```python
from build123d import *

# Parameters (mm, degrees)
BOSS_EXTRUDE1_DEPTH = 6.35
SKETCH2_W           = 71.12
SKETCH2_H           = 9.525
CUT_EXTRUDE1_DEPTH  = 223.34069578
SKETCH3_W           = 9.652
SKETCH3_H           = 38.1
SKETCH3_W_2         = 9.62146782
CUT_EXTRUDE2_DEPTH  = 6.35


with BuildPart() as part:
    # Sketch1 → Boss-Extrude1 (new body)
    with BuildSketch(Plane(origin=(0, 0, 0), x_dir=(1, 0, 0), z_dir=(0, 1, 0))):
        Polygon((-177.8, -7.239), (-177.8, 42.672), (-87.122, 133.35), (87.122, 133.35), (177.8, 42.672), (177.8, -7.239), (168.275, -7.239), (168.275, -83.439), (177.8, -83.439), (177.8, -133.35), (76.2, -133.35), (76.2, -123.825), (-76.2, -123.825), (-76.2, -133.35), (-177.8, -133.35), (-177.8, -83.439), (-168.275, -83.439), (-168.275, -7.239), align=None)
    extrude(amount=BOSS_EXTRUDE1_DEPTH)

    # Sketch2 → Cut-Extrude1 (cut, through all)
    with BuildSketch(Plane(origin=(0, 6.35, 0), x_dir=(1, 0, 0), z_dir=(0, 1, 0))):
        with Locations((71.12, 36.5125)):
            Rectangle(SKETCH2_W, SKETCH2_H)
        with Locations((-71.12, 36.5125)):
            Rectangle(SKETCH2_W, SKETCH2_H)
    extrude(amount=-CUT_EXTRUDE1_DEPTH, mode=Mode.SUBTRACT)

    # Sketch3 → Cut-Extrude2 (cut)
    with BuildSketch(Plane(origin=(0, 6.35, 0), x_dir=(1, 0, 0), z_dir=(0, 1, 0))):
        with Locations((75.702840569, 89.027)):
            Rectangle(SKETCH3_W, SKETCH3_H)
        with Locations((-75.596992051, 89.027)):
            Rectangle(SKETCH3_W_2, SKETCH3_H)
    extrude(amount=-CUT_EXTRUDE2_DEPTH, mode=Mode.SUBTRACT)


solid = part.part
```
Design review of the part built by this model. Coordinates are the model's own, in mm. Give positions to 0.01 mm unless a question says otherwise; leave off trailing zeros. Order: outer loops, then holes, each group sorted by start corner. A loop starts at its lowest first (then second) coordinate and runs counter-clockwise, first axis right, second up. Notation, with made-up numbers: (47.5, -20) -> (90.5, -20) arc R9 ccw to (90.5, -6) -> close; hole circle Ø9 at (-27, -13.75). An arc over 180 degrees is marked (long way). Write item = value, one per line. Start each with the question number.
(1) We need section A-A on x = 57. Write out the cut boundary in (y, z) (3 decimals), plus the area to 3 significant figures.
(2) To check wall thickness, follow line 1 along X through (y, z) = (2, -99); line 2 along Z through (x, y) = (70.5, 5.5) (3 decimals); line 3 along X through (y, z) = (3.25, -38.5). State the ranges of each line that lie inside material, in increasing order.
(3) We need section B-B on y = 1. State how many separate pieces and enclosed holes the cut face has, plus the area to 3 significant figures.
(4) For pin 1 (1 mm diameter, centred on y = 2, z = -66.5, fed in from -X); pin 2 (2 mm diameter, centred on y = 5, z = 8.5, fed in from +X) (3 decimals); pin 3 (1.9 mm diameter, centred on x = 75, y = 4.5, fed in from +Z) (3 decimals), all flat-tipped, find the tip position at first contact; note any pin that passes through.
(5) We need section D-D on x = -150.5. Write out the cut boundary in (y, z).
(6) We need section C-C on z = 11.5. Write out the cut boundary in (x, y) (3 decimals), plus the area to 3 significant figures.
Numbers:
q1.outline = (0, -133.35) -> (6.35, -133.35) -> (6.35, -41.275) -> (0, -41.275) -> close; (0, -31.75) -> (6.35, -31.75) -> (6.35, 123.825) -> (0, 123.825) -> close
q1.area = 1,570 mm^2
q2.line_1 = -121.47 to -80.41, -70.79 to 70.88, 80.53 to 121.47
q2.line_2 = -133.35 to -41.275, -31.75 to 123.825
q2.line_3 = -177.8 to -106.68, -35.56 to 35.56, 106.68 to 177.8
q3.separate_pieces = 1
q3.enclosed_holes = 4
q3.area = 81,600 mm^2
q4.pin_1 = -154.47
q4.pin_2 = 168.275
q4.pin_3 = 123.825
q5.outline = (0, -69.97) -> (6.35, -69.97) -> (6.35, 133.35) -> (0, 133.35) -> close
q6.outline = (-168.275, 0) -> (168.275, 0) -> (168.275, 6.35) -> (-168.275, 6.35) -> close
q6.area = 2,140 mm^2
